from build123d import *

# Parameters (mm, degrees)
SKETCH_W    = 160
SKETCH_H    = 75
PAD_DEPTH   = 5
SKETCH001_R = 2.25
HOLE_DEPTH  = 5.001


with BuildPart() as part:
    # Sketch → Pad (new body)
    with BuildSketch(Plane.XY):
        Rectangle(SKETCH_W, SKETCH_H)
    extrude(amount=PAD_DEPTH)

    # Sketch001 (on Face5 of Pad) → Hole (cut, through all)
    with BuildSketch(Plane(origin=(0, 0, 0), x_dir=(1, 0, 0), z_dir=(0, 0, -1))):
        with Locations((-75, 32.5)):
            Circle(SKETCH001_R)
        with Locations((75, 32.5)):
            Circle(SKETCH001_R)
        with Locations((75, -32.5)):
            Circle(SKETCH001_R)
        with Locations((-75, -32.5)):
            Circle(SKETCH001_R)
    extrude(amount=-HOLE_DEPTH, mode=Mode.SUBTRACT)


solid = part.part
Check sheet for the modelled part. Datum: model origin and axes. Units: mm. Give positions to 0.01 mm unless a question says otherwise; leave off trailing zeros. Loops run counter-clockwise (first coordinate to the right, second up) from the corner with the lowest first, then second, coordinate; pieces in that order, holes last. Notation, with made-up numbers: M 78,77.25 L 107,77.25 A26 cw 107,99.25 Z; hole C 36,27 d7. An arc over 180 degrees is marked long. Answer as a JSON object with one key per item and string values. Group by question number.
Q1. Cross-section at B-B on y = -32.5. Record the cut outline in (x, z), then the cut area to 3 significant figures.
Q2. Go/stop test with a flat-tipped pin: P1, Ø2.5, axis at x = -75, y = -32.5, coming from the -Z side. Record where the tip stops, or that it passes through.
Q3. Cross-section at A-A on x = -75. Record the cut outline in (y, z).
Q4. Release check for a two-part mould opening along Y. For faces 1 (the cylindrical face through (-73.79, 30.603, 2.465)), 2 (the flat face through (-1, 37.5, 2)), 3 (the flat face through (-80, -1, 2)) record: released by +Y, released by -Y, zero draft, split by the parting line, or undercut.
Q5. Material ranges on line 1 along Y through (x, z) = (-75, 3.1); line 2 along X through (y, z) = (32.5, 2.9); line 3 along X through (y, z) = (30.5, 4.7), recorded low to high. Write a range as [from, to].
Evaluation:
{
 "1": {"outline": "M -80,0 L -77.25,0 L -77.25,5 L -80,5 Z; M -72.75,0 L 72.75,0 L 72.75,5 L -72.75,5 Z; M 77.25,0 L 80,0 L 80,5 L 77.25,5 Z", "area": "755 mm2"},
 "2": {"P1": "passes through"},
 "3": {"outline": "M -37.5,0 L -34.75,0 L -34.75,5 L -37.5,5 Z; M -30.25,0 L 30.25,0 L 30.25,5 L -30.25,5 Z; M 34.75,0 L 37.5,0 L 37.5,5 L 34.75,5 Z"},
 "4": {"face 1": "undercut", "face 2": "released by +Y", "face 3": "zero draft"},
 "5": {"line 1": "y = [-37.5, -34.75], [-30.25, 30.25], [34.75, 37.5]", "line 2": "x = [-80, -77.25], [-72.75, 72.75], [77.25, 80]", "line 3": "x = [-80, -76.03], [-73.97, 73.97], [76.03, 80]"}
}
